Autodesk Inventor part; units mm, degrees
ref_plane "YZ Plane" through (0, 0, 0) normal (1, 0, 0) x (0, 1, 0)
ref_plane "XZ Plane" through (0, 0, 0) normal (0, 1, 0) x (-1, 0, 0)
ref_plane "XY Plane" through (0, 0, 0) normal (0, 0, 1) x (1, 0, 0)
sketch "スケッチ1" plane through (0, 0, 0) normal (0, 0, 1) x (1, 0, 0)
  circle A0 centre (0, 0) radius 65 construction
  line L0 (-42.5, 65) -> (42.5, 65) construction
  line L1 (42.5, 65) -> (42.5, -65) construction
  line L2 (42.5, -65) -> (-42.5, -65) construction
  line L3 (-42.5, -65) -> (-42.5, 65) construction
  arc A1 (42.5, 49.1808) -> (-42.5, 49.1808) centre (0, 0) ccw
  line L4 (-42.5, 49.1808) -> (-42.5, -49.1808)
  line L5 (42.5, 49.1808) -> (42.5, -49.1808)
  arc A2 (-42.5, -49.1808) -> (42.5, -49.1808) centre (0, 0) ccw
  point P0 (0, 65)
  dimension "d0" = 130
  dimension "d1" = 85
extrude "基板" add sketch "スケッチ1" along normal blind 1.6
sketch "スケッチ4" plane through (0, 0, 1.6) normal (0, 0, 1) x (1, 0, 0)
  line L0 (0, -55.1622) -> (0, 55.1622) construction
  line L1 (42.5, -49.1808) -> (42.5, 49.1808) construction
  circle A0 centre (0, 0) radius 60 construction
  line L2 (0, 0) -> (36.3616, 43.334) construction
  line L3 (0, 0) -> (56.5685, 0) construction
  point P0 (38.5, -46.019)
  point P1 (-38.5, -46.019)
  point P2 (38.5673, 45.9627)
  point P3 (-38.5673, 45.9627)
  dimension "d27" = 4
  dimension "d29" = 120
  dimension "d30" = 50
hole "スペーサ取付穴" at (38.5, -46.019, 1.6) at (-38.5, -46.019, 1.6) at (38.5673, 45.9627, 1.6) at (-38.5673, 45.9627, 1.6) direction (0, 0, -1) diameter 3.2 end through all
sketch "スケッチ5" plane through (0, 0, 1.6) normal (0, 0, 1) x (1, 0, 0)
  line L0 (-30, -12) -> (30, -12)
  line L1 (30, -12) -> (30, -30)
  line L2 (30, -30) -> (-30, -30)
  line L3 (-30, -30) -> (-30, -12)
  point P0 (0, 0)
  point P1 (0, -12)
  dimension "d38" = 60
  dimension "d39" = 18
  dimension "d40" = 12
extrude "バッテリー通し穴" cut sketch "スケッチ5" against normal through all
properties part number "BaseBoard2"
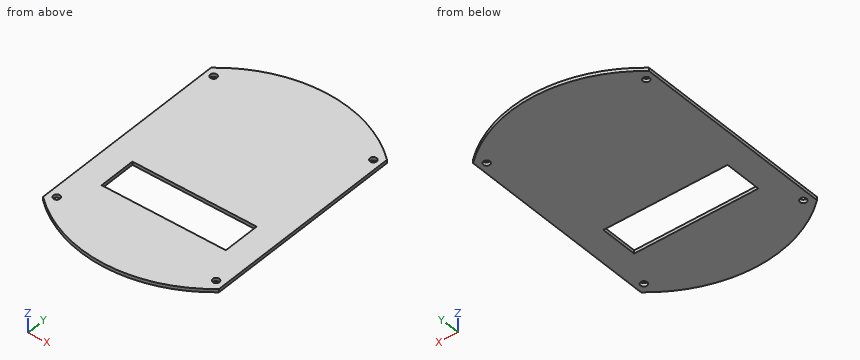
Read the model definition and answer for the solid it produces. Units are mm, in the model's axes. Coordinates: 2 decimals unless noted, no trailing zeros. Loops run counter-clockwise (first coordinate to the right, second up) from the corner with the lowest first, then second, coordinate; pieces in that order, holes last. Notation, with made-up numbers: (88, 77.5) -> (101, 77.5) arc R25 cw to (101, 107.5) -> close; hole circle Ø5 at (-21, 38.25). An arc over 180 degrees is marked (long way). Write item = value, one per line. Start each with the question number.
1) The part is cut by section C-C, the plane z = 1.1. Determine the outline of the cut face in (x, y), plus the area to 3 significant figures.
2) The part is cut by section D-D, the plane x = 33. Determine the outline of the cut face in (y, z).
3) Find the intervals of material crossed by L1, parallel to Y at x = 38.5, z = 0.7; L2, parallel to X at y = -22, z = 0.45; L3, parallel to Y at x = 27.5, z = 0.1, in increasing order. Write a range as from..to.
4) Given P1, Ø0.5, axis at x = -11, z = 1, coming from the +Y side; P2, Ø3.5, axis at x = -38.57, y = 45.96, coming from the -Z side; P3, Ø0.8, axis at x = -3, z = 0.5, coming from the -Y side, each flat-ended and moving along its own axis, determine where each tip first touches the part or whether it passes through.
5) The part is cut by section B-B, the plane x = -19. Determine the outline of the cut face in (y, z), plus the area to 3 significant figures.
6) The part is cut by section A-A, the plane y = -22.5. Determine the outline of the cut face in (x, z).
Result:
q1.outline = (-42.5, -49.18) arc R65 ccw to (42.5, -49.18) -> (42.5, 49.18) arc R65 ccw to (-42.5, 49.18) -> close; hole circle Ø3.2 at (-38.57, 45.96); hole circle Ø3.2 at (-38.5, -46.02); hole (-30, -30) -> (30, -30) -> (30, -12) -> (-30, -12) -> close; hole circle Ø3.2 at (38.5, -46.02); hole circle Ø3.2 at (38.57, 45.96)
q1.area = 9,090 mm²
q2.outline = (-56, 0) -> (56, 0) -> (56, 1.6) -> (-56, 1.6) -> close
q3.L1 = -52.37..-47.62, -44.42..44.36, 47.56..52.37
q3.L2 = -42.5..-30, 30..42.5
q3.L3 = -58.9..-30, -12..58.9
q4.P1 = 64.1
q4.P2 = 0
q4.P3 = -64.95
q5.outline = (-62.16, 0) -> (-30, 0) -> (-30, 1.6) -> (-62.16, 1.6) -> close; (-12, 0) -> (62.16, 0) -> (62.16, 1.6) -> (-12, 1.6) -> close
q5.area = 170 mm²
q6.outline = (-42.5, 0) -> (-30, 0) -> (-30, 1.6) -> (-42.5, 1.6) -> close; (30, 0) -> (42.5, 0) -> (42.5, 1.6) -> (30, 1.6) -> close
